Source: CAD feature listing. Evaluate the final solid. Frame: model axes, mm. Face numbers are marked on the shaded views. Coordinates: 2 decimals unless noted, no trailing zeros. Loops run counter-clockwise (first coordinate to the right, second up) from the corner with the lowest first, then second, coordinate; pieces in that order, holes last.
```python
from build123d import *

# Parameters (mm, degrees)
CYLINDER001_R     = 27.5
CYLINDER001_DEPTH = 6
CYLINDER_R        = 20.75
CYLINDER_DEPTH    = 12


with BuildPart() as cylinder001:
    # Cylinder001 → Cylinder001 (new body)
    with BuildSketch(Plane.XY.offset(12)):
        Circle(CYLINDER001_R)
    extrude(amount=CYLINDER001_DEPTH)


with BuildPart() as cone:
    # Cone → Cone (revolve)
    with BuildSketch(Plane(origin=(0, 0, 18), x_dir=(1, 0, 0), z_dir=(0, -1, 0))):
        Polygon((0, 0), (11, 0), (13, 8), (0, 8), align=None)
    revolve(axis=Axis((0, 0, 18), (0, 0, 1)))


with BuildPart() as viewfinder_port:
    # Cylinder → Cylinder (new body)
    with BuildSketch(Plane.XY):
        Circle(CYLINDER_R)
    extrude(amount=CYLINDER_DEPTH)

    # Fusion: union Cylinder001, Cone
    add(cylinder001.part)
    add(cone.part)


solid = viewfinder_port.part
```
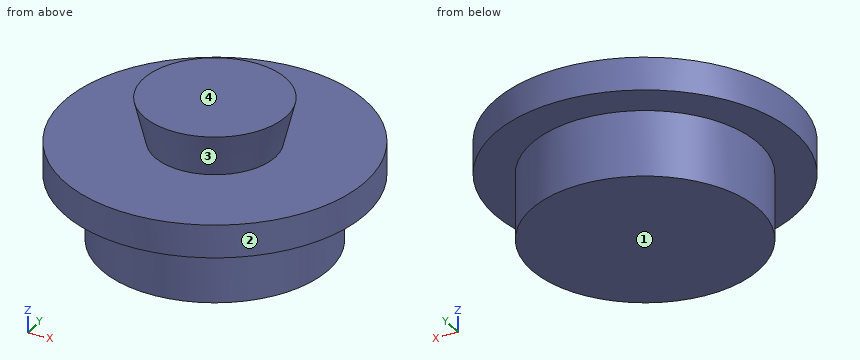
Q1. Material intervals for line 1 along Z through (x, y) = (20, -18); line 2 along Z through (x, y) = (19.5, -6); line 3 along X through (y, z) = (-1.5, 18.5), sorted ascending.
Q2. Section query C-C on z = 16.25. Return the cut outline in (x, y).
Q3. Section query A-A on y = 0. Return the cut outline in (x, z).
Q4. Section query D-D on y = 16. Return the cut outline in (x, z), then the cut area to 3 significant figures.
Q5. First-contact query: pin 1 Ø12 at (x, y) = (7.5, -18) entering from -Z; pin 2 Ø6 at (x, z) = (-13, 15.5) entering from -Y; pin 3 Ø1 at (x, z) = (0, 21) entering from +Y (3 decimals); pin 4 Ø5 at (y, z) = (18, 19) entering from -X. Flat tips, straight axial feed; report the tip coordinate or a pass-through.
Q6. Draft query along Z for the marked faces 1, 2, 3 and 4. Return one class per face: released by +Z, released by -Z, zero draft, split by the parting line, or undercut.
Resolved:
1. line 1: z = 12 to 18
1. line 2: z = 0 to 18
1. line 3: x = -11.02 to 11.02
2. outline: circle Ø55 at (0, 0)
3. outline: (-27.5, 12) - (-20.75, 12) - (-20.75, 0) - (20.75, 0) - (20.75, 12) - (27.5, 12) - (27.5, 18) - (11, 18) - (13, 26) - (-13, 26) - (-11, 18) - (-27.5, 18) - close
4. outline: (-22.37, 12) - (-13.21, 12) - (-13.21, 0) - (13.21, 0) - (13.21, 12) - (22.37, 12) - (22.37, 18) - (-22.37, 18) - close
4. area: 585 mm2
5. pin 1: stops at z = 0
5. pin 2: stops at y = -25.62
5. pin 3: stops at y = 11.875
5. pin 4: stops at x = -22.57
6. face 1: released by -Z
6. face 2: zero draft
6. face 3: undercut
6. face 4: released by +Z
